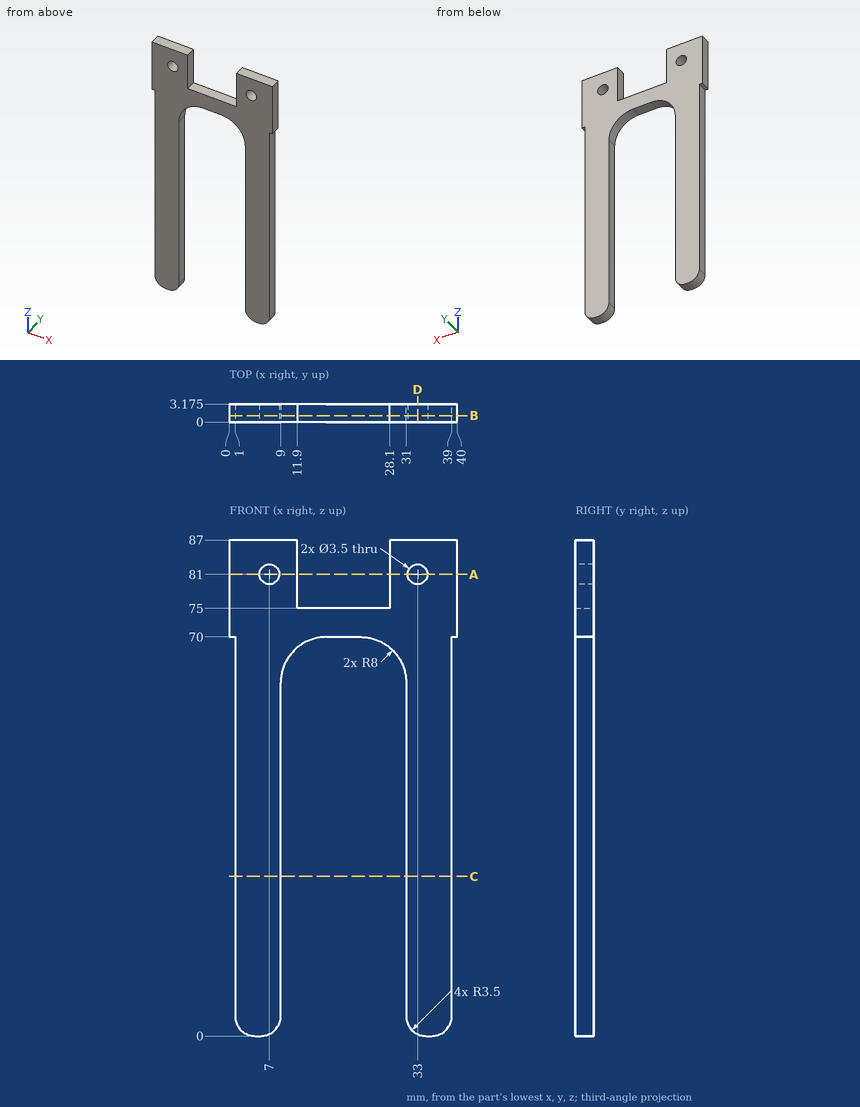
Could you check a few things on this drawing? It's one solid part, dimensions in mm from its lowest x, y, z. Give positions to 0.01 mm unless a question says otherwise; leave off trailing zeros. Order: outer loops, then holes, each group sorted by start corner. A loop starts at its lowest first (then second) coordinate and runs counter-clockwise, first axis right, second up. Notation, with made-up numbers: (41, -11.75) - (81, -11.75) arc R23 ccw to (81, 5.25) - close; hole circle Ø1 at (-4.5, -1.5). An arc over 180 degrees is marked (long way). One line per item, written item: value. Start each with the question number.
1. For P1, Ø1.6, axis at y = 1, z = 36, coming from the +X side; P2, Ø1.6, axis at y = 1.5, z = 79.5, coming from the -X side; P3, Ø1.6, axis at y = 1, z = 30.5, coming from the -X side, each with a flat end and sliding along its axis, tell me the tip position at first contact or that it passes through.
2. Imagine slicing it at B-B on y = 1.15. List the corners of the cut face in (x, z) for me.
3. Imagine slicing it at D-D on x = 33. List the corners of the cut face in (y, z) for me (3 decimals), plus the area to 3 significant figures.
4. If I drill on probe 1 along X at (y, z) = (2.3, 81); probe 2 along X at (y, z) = (2.7, 29.5); probe 3 along X at (y, z) = (2.2, 78.5), over which ranges is the centre line in solid material (lowest first)?
5. Imagine slicing it at C-C on z = 28. List the corners of the cut face in (x, y) for me (3 decimals), plus the area to 3 significant figures.
6. Imagine slicing it at A-A on z = 81. List the corners of the cut face in (x, y) for me (3 decimals), plus the area to 3 significant figures.
Values:
1. P1: x = 39
1. P2: x = 0
1. P3: x = 1
2. outline: (0, 70) - (1, 70) - (1, 3.5) arc R3.5 ccw to (4.5, 0) - (5.5, 0) arc R3.5 ccw to (9, 3.5) - (9, 62) arc R8 cw to (17, 70) - (23, 70) arc R8 cw to (31, 62) - (31, 3.5) arc R3.5 ccw to (34.5, 0) - (35.5, 0) arc R3.5 ccw to (39, 3.5) - (39, 70) - (40, 70) - (40, 87) - (28.1, 87) - (28.1, 75) - (11.9, 75) - (11.9, 87) - (0, 87) - close; hole circle Ø3.5 at (7, 81); hole circle Ø3.5 at (33, 81)
3. outline: (0, 0.338) - (3.175, 0.338) - (3.175, 79.25) - (0, 79.25) - close; (0, 82.75) - (3.175, 82.75) - (3.175, 87) - (0, 87) - close
3. area: 264 mm²
4. probe 1: 0 to 5.25, 8.75 to 11.9, 28.1 to 31.25, 34.75 to 40
4. probe 2: 1 to 9, 31 to 39
4. probe 3: 0 to 11.9, 28.1 to 40
5. outline: (1, 0) - (9, 0) - (9, 3.175) - (1, 3.175) - close; (31, 0) - (39, 0) - (39, 3.175) - (31, 3.175) - close
5. area: 50.8 mm²
6. outline: (0, 0) - (5.25, 0) - (5.25, 3.175) - (0, 3.175) - close; (8.75, 0) - (11.9, 0) - (11.9, 3.175) - (8.75, 3.175) - close; (28.1, 0) - (31.25, 0) - (31.25, 3.175) - (28.1, 3.175) - close; (34.75, 0) - (40, 0) - (40, 3.175) - (34.75, 3.175) - close
6. area: 53.3 mm²
